Build history of the part. All positions in model axes, mm. Face numbers are marked on the shaded views. Round coordinates to 2 decimals unless told otherwise and drop trailing zeros. Loops run counter-clockwise (first coordinate to the right, second up) from the corner with the lowest first, then second, coordinate; pieces in that order, holes last.
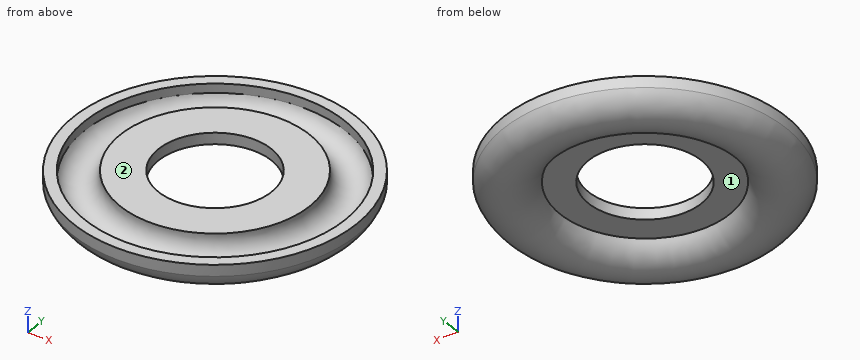
from build123d import *

# Parameters (mm, degrees)
SKETCH_1_R               = 12.5
EXTRUDE_1_DEPTH          = 1
CUT_EXTRUDE_1_DEPTH      = 18.767490446
CUT_EXTRUDE_1_DEPTH_BACK = 18.767490446
SKETCH_4_R               = 5


# Read off the part's stored shape, not the designer's step: 抽壳1
with BuildPart() as part:
    # 草图1 → 凸台-拉伸1 (new body)
    with BuildSketch(Plane.XY):
        Circle(SKETCH_1_R)
    extrude(amount=EXTRUDE_1_DEPTH)

    # 扫描1: sweep along a path in 草图2
    with BuildLine(Plane(origin=(0, 0, 0), x_dir=(-1, 0, 0), z_dir=(0, 0, -1))) as sweep_1_path:
        CenterArc((0, 0), 12.5, 0, 360)
    # 草图3 → 扫描1 (sweep)
    with BuildSketch(Plane(origin=(0, 0, 0), x_dir=(1, 0, 0), z_dir=(0, 1, 0))):
        with BuildLine():
            Line((-12.5, 0), (-7.5, 0))
            ThreePointArc((-7.5, 0), (-10, 1.784295774), (-12.5, 0))
        make_face()
    sweep(path=sweep_1_path.line)

    # 抽壳1 outline → 抽壳1 (revolve, cut)
    with BuildSketch(Plane.XZ):
        with BuildLine():
            Line((11.5, 0.18751359), (11.5, 1))
            Line((11.5, 1), (8.362499328, 1))
            ThreePointArc((8.362499328, 1), (9.587980401, -0.731813124), (11.5, 0.18751359))
        make_face()
    revolve(axis=Axis((0, 0, 0), (0, 0, 1)), mode=Mode.SUBTRACT)

    # 草图4 → 切除-拉伸1 (cut, two sides: drawn at the far end of the back side and taken through both)
    with BuildSketch(Plane(origin=(0, 0, 0), x_dir=(-1, 0, 0), z_dir=(0, 0, -1)).offset(-CUT_EXTRUDE_1_DEPTH_BACK)):
        Circle(SKETCH_4_R)
    extrude(amount=CUT_EXTRUDE_1_DEPTH + CUT_EXTRUDE_1_DEPTH_BACK, mode=Mode.SUBTRACT)


solid = part.part
(1) Pull direction X, two halves, no side cores. Call the marked faces 1 and 2: +X half, -X half, draft (parallel to the pull), parting line (faces both ways), or undercut.
Responses:
face 1: undercut
face 2: draft
(2) Pin check, flat tips, straight feed: P1, Ø12, axis at x = 0.5, y = -1.5, coming from the -Z side; P2, Ø1.5, axis at x = -0.5, y = -4.5, coming from the -Z side; P3, Ø6, axis at x = 0, y = 0, coming from the -Z side; P4, Ø1.5, axis at x = -1.5, z = -0.5, coming from the -Y side. Stop position of each tip, or through.
Responses:
P1: stops at z = -0.21
P2: stops at z = 0
P3: passes through
P4: stops at y = -12.46
(3) Slice it at C-C on z = -1.2. List the corners of the cut face in (x, y), plus the area to 3 significant figures.
Responses:
outline: circle Ø23.32 at (0, 0); hole circle Ø16.68 at (0, 0)
area: 208 mm2
(4) Probe line 1 (Y direction, x = 0, z = 0.7); line 2 (X direction, y = 1, z = 0.1); line 3 (Y direction, x = -3.25, z = 0.85). List the from-to ranges inside material, lowest first.
Responses:
line 1: y = -12.5 to -11.5, -8.36 to -5, 5 to 8.36, 11.5 to 12.5
line 2: x = -12.46 to -11.41, -8.48 to -4.9, 4.9 to 8.48, 11.41 to 12.46
line 3: y = -12.07 to -11.03, -7.7 to -3.8, 3.8 to 7.7, 11.03 to 12.07
(5) Slice it at A-A on x = 0. List the corners of the cut face in (y, z).
Responses:
outline: (-12.5, 0) arc R2.64 ccw to (-7.5, 0) - (-5, 0) - (-5, 1) - (-8.36, 1) arc R1.64 cw to (-11.5, 0.19) - (-11.5, 1) - (-12.5, 1) - close; (5, 0) - (7.5, 0) arc R2.64 ccw to (12.5, 0) - (12.5, 1) - (11.5, 1) - (11.5, 0.19) arc R1.64 cw to (8.36, 1) - (5, 1) - close
